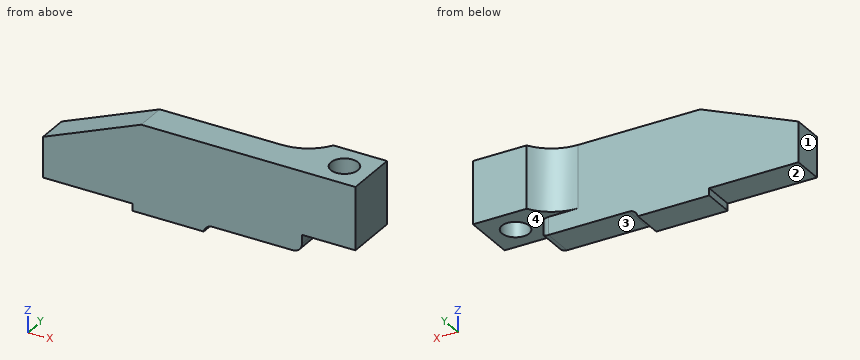
from build123d import *

# Parameters (mm, degrees)
EXTRUDE_1_DEPTH     = 3.5
SKETCH_2_W          = 6
SKETCH_2_H          = 9
EXTRUDE_2_DEPTH     = 5.95
SKETCH_3_R          = 1.525
CUT_EXTRUDE_1_DEPTH = 38.475358571
SKETCH_4_W          = 8
SKETCH_4_H          = 2.2
CUT_EXTRUDE_2_DEPTH = 10
CUT_EXTRUDE_START   = -9
SKETCH_5_W          = 6
SKETCH_5_H          = 5.95
CUT_EXTRUDE_4_DEPTH = 2
FILLET_1_R          = 5
FILLET_2_R          = 1
FILLET_3_R          = 1


with BuildPart() as part:
    # 草图1 → 凸台-拉伸1 (new body)
    with BuildSketch(Plane(origin=(0, 0, 0), x_dir=(1, 0, 0), z_dir=(0, 1, 0))):
        Polygon((0, 0), (0, 9), (-17, 9), (-17, 12), (-24, 12), (-25, 12), (-25, 9), (-34, 9), (-35, 9), (-35, 4.5), (-24, 0), (-8, 0), align=None)
    extrude(amount=EXTRUDE_1_DEPTH)

    # 草图2 → 凸台-拉伸2 (add)
    with BuildSketch(Plane(origin=(0, 0, 0), x_dir=(1, 0, 0), z_dir=(0, 1, 0))):
        with Locations((-3, 4.5)):
            Rectangle(SKETCH_2_W, SKETCH_2_H)
    extrude(amount=EXTRUDE_2_DEPTH)

    # 草图3 → 切除-拉伸1 (cut, through all)
    with BuildSketch(Plane.XY):
        with Locations((-3, 2.975)):
            Circle(SKETCH_3_R)
    extrude(amount=-CUT_EXTRUDE_1_DEPTH, mode=Mode.SUBTRACT)

    # 草图4 → 切除-拉伸2 (cut)
    with BuildSketch(Plane(origin=(0, 0, 0), x_dir=(1, 0, 0), z_dir=(0, 1, 0))):
        with Locations((-21, 10.9)):
            Rectangle(SKETCH_4_W, SKETCH_4_H)
    extrude(amount=CUT_EXTRUDE_2_DEPTH, mode=Mode.SUBTRACT)

    # 草图5 → 切除-拉伸4 (cut)
    with BuildSketch(Plane.XY.offset(CUT_EXTRUDE_START)):
        with Locations((-3, 2.975)):
            Rectangle(SKETCH_5_W, SKETCH_5_H)
    extrude(amount=CUT_EXTRUDE_4_DEPTH, mode=Mode.SUBTRACT)

    # 圆角1
    # the kernel refuses this fillet: 5 mm, written as the material it adds along each edge
    with BuildSketch(Plane(origin=(-6, 3.5, -7), x_dir=(-1, 0, 0), z_dir=(0, 0, 1))) as fillet_1_piece_1:
        with BuildLine():
            CenterArc((4.300872005, -5), FILLET_1_R, 90, 59.336170258)
            Line((0, -2.45), (0, 0))
            Line((0, 0), (4.300872005, 0))
        make_face()
    extrude(amount=7)

    # 圆角2
    fillet_2_edges = [part.edges().sort_by_distance(p)[0] for p in [
        (-6, 3.5, -8),
        (-6, 1.75, -9),
    ]]
    fillet(fillet_2_edges, radius=FILLET_2_R)

    # 圆角3
    # the kernel refuses this fillet: 1 mm, written as the material it adds along each edge
    with BuildSketch(Plane(origin=(-17, 0, -9), x_dir=(1, 0, 0), z_dir=(0, 1, 0))) as fillet_3_piece_1:
        with BuildLine():
            CenterArc((0.979795897, 1), FILLET_3_R, 191.536959033, 78.463040967)
            Line((0, 0.8), (-0.019595918, 0.796))
            ThreePointArc((-0.019595918, 0.796), (-0.02, 0.4), (-0.02, 0))
            Line((-0.02, 0), (0, -0.02))
            Line((0, -0.02), (0.979795897, -0.02))
            Line((0.979795897, -0.02), (0.979795897, 0))
        make_face()
    extrude(amount=3.5)


solid = part.part
Work out the finished part from the listing and answer in its coordinate system (mm). Face numbers are marked on the shaded views. A direction names the side the tool comes from. Round coordinates to 2 decimals unless told otherwise and drop trailing zeros. Order: outer loops, then holes, each group sorted by start corner. A loop starts at its lowest first (then second) coordinate and runs counter-clockwise, first axis right, second up. Notation, with made-up numbers: M 51.5,77.25 L 58.5,77.25 A24 cw 58.5,108.25 Z; hole C 10.5,-8 d10. An arc over 180 degrees is marked long. One line per item, written item: value.
Q1. Find section C-C on z = -7.5. Write down the section's boundary in (x, y), then the cut area to 3 significant figures.
Derived:
outline: M -35,0 L -6,0 L -6,2.5 A1 ccw -7,3.5 L -35,3.5 Z
area: 101 mm²
Q2. Find section B-B on y = 0.7. Write down the section's boundary in (x, z).
Derived:
outline: M -35,-9 L -25,-9 L -25,-9.8 L -17,-9.8 A1 cw -16.02,-9 L -7,-9 A1 ccw -6,-8 L -6,-7 L 0,-7 L 0,0 L -24,0 L -35,-4.5 Z
Q3. Find section D-D on x = -15.5. Write down the section's boundary in (y, z), then the cut area to 3 significant figures.
Derived:
outline: M 0,-9 L 3.5,-9 L 3.5,0 L 0,0 Z
area: 31.5 mm²
Q4. Straight lines are drawn through the part: line 1 (Y direction, x = -3, z = -3); line 2 (Z direction, x = -4.5, y = 0.5); line 3 (Y direction, x = -30.5, z = -5.25). For each, find the intervals that lie inside material, in ascending order.
Derived:
line 1: 0 to 1.45, 4.5 to 5.95
line 2: -7 to 0
line 3: 0 to 3.5
Q5. For the marked faces 1, 2, 3 and 4, determine the directions among +Z, -Z, +X, -X, +Y, -Y from which every point of the face is accessible in a straight line to the end or side of a thin tool.
Derived:
face 1: +Z, -Z, -X, +Y, -Y
face 2: -Z, -X, +Y, -Y
face 3: -Z, +X, +Y, -Y
face 4: -Z, +X, +Y
Q6. Find section A-A on x = -3. Write down the section's boundary in (y, z).
Derived:
outline: M 0,-7 L 1.45,-7 L 1.45,0 L 0,0 Z; M 4.5,-7 L 5.95,-7 L 5.95,0 L 4.5,0 Z
Q7. Flat-ended cylindrical pins translate along their axes: pin 1 (4 mm diameter, centred on x = -22, z = -2, fed in from +Y); pin 2 (2 mm diameter, centred on x = -10, y = 1.5, fed in from -Z); pin 3 (1.8 mm diameter, centred on x = -3, y = 2.975, fed in from -Z). Find the tip coordinate at first contact, or state that the pin passes through.
Derived:
pin 1: y = 3.5
pin 2: z = -9
pin 3: through
